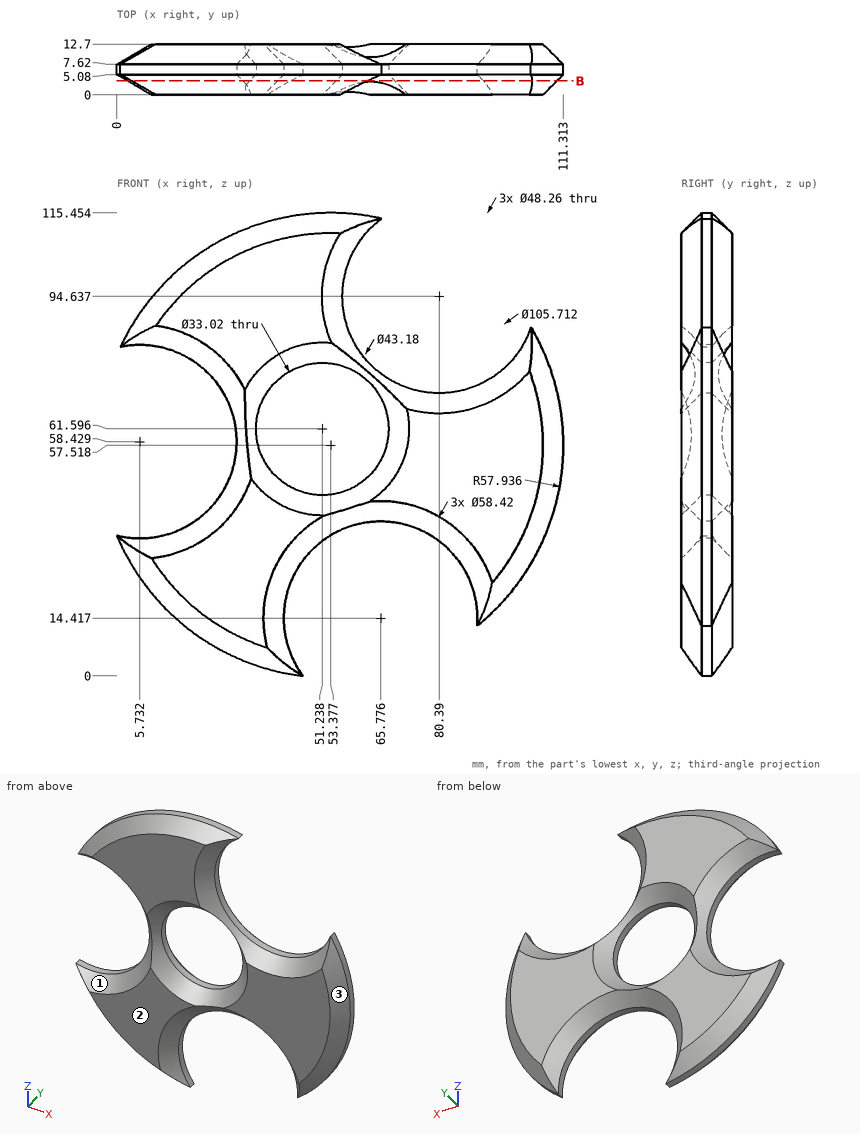
Could you check a few things on this drawing? It's one solid part, dimensions in mm from its lowest x, y, z. Round coordinates to 2 decimals unless told otherwise and drop trailing zeros. Order: outer loops, then holes, each group sorted by start corner. A loop starts at its lowest first (then second) coordinate and runs counter-clockwise, first axis right, second up. Notation, with made-up numbers: M 72.5,19.5 L 129.5,19.5 A16 ccw 129.5,27.5 Z; hole C -18.75,-24 d1. An arc over 180 degrees is marked long. One line per item, written item: value.
(1) If we mould it in two halves opening along Z, with no side actions, what happens to the marked faces 1, 2 and 3? For each: released by +Z, released by -Z, zero draft, split by the parting line, or undercut.
Ans:
face 1: undercut
face 2: zero draft
face 3: split by the parting line
(2) I need wall thicknesses on line 1 along X through (y, z) = (11.5, 23) (1 decimal); line 2 along X through (y, z) = (5.75, 62.5) (1 decimal); line 3 along Z through (x, y) = (51.5, 4) (1 decimal). Which ranges of each line are inside material? Lowest first, please. Write a range as from..to.
Ans:
line 1: x = 11.8..39.1, 92.4..95
line 2: x = 29.5..34.8, 67.7..111.1
line 3: z = 35.2..44, 79.2..114.3
(3) I'm going to push flat-ended pins straight in: P1, Ø12, axis at x = 59.5, z = 56, coming from the +Y side; P2, Ø6, axis at x = 59.5, y = 6, coming from the -Z side; P3, Ø10, axis at x = 35, z = 58.5, coming from the -Y side; P4, Ø2, axis at x = 48.5, z = 42, coming from the +Y side (1 decimal). Where does each tip first touch, or does it pass through?
Ans:
P1: passes through
P2: stops at z = 36.69
P3: stops at y = 1.71
P4: stops at y = 11.9
(4) Imagine slicing it at B-B (y = 3.5). Write out the boundary of the cut face in (x, z) (1 decimal).
Ans:
outline: M 2.7,32.9 A56.4 ccw 43.2,2.1 A25.7 cw long 91.4,16 A56.4 ccw 103.5,83.3 A25.7 cw long 62.5,113.1 A56.4 ccw 3.7,84.1 A25.7 cw long Z; hole C 51.2,61.6 d36.2
